Work out the finished part from the listing and answer in its coordinate system (mm). A direction names the side the tool comes from. Give positions to 0.01 mm unless a question says otherwise; leave off trailing zeros. Order: outer loops, then holes, each group sorted by start corner. A loop starts at its lowest first (then second) coordinate and runs counter-clockwise, first axis right, second up. Notation, with made-up numbers: (73, 72) -> (128, 72) arc R19 cw to (128, 92) -> close; hole circle Ø9 at (19, 58). An arc over 180 degrees is marked (long way). Use a Markdown table: item, result. Add a question column.
```python
from build123d import *

# Parameters (mm, degrees)
SKETCH_1_R            = 13.5
EXTRUDE_1_DEPTH       = 8
SKETCH_7_W            = 34
SKETCH_7_H            = 30
SKETCH_7_R            = 13.5
EXTRUDE_2_DEPTH       = 8
SKETCH_11_W           = 5
SKETCH_11_H           = 30
EXTRUDE_6_DEPTH       = 40
FILLET_2_R            = 10
SKETCH_13_R           = 8.5
SKETCH_13_R_2         = 7.5
CUT_EXTRUDE_3_DEPTH   = 2.5
SKETCH_14_R           = 3.5
CUT_EXTRUDE_4_DEPTH   = 36
SKETCH_22_W           = 41
SKETCH_22_H           = 5
EXTRUDE_8_DEPTH       = 8
SKETCH_23_W           = 12
SKETCH_23_H           = 8
CUT_EXTRUDE_6_DEPTH   = 20
RIB_1_REACH           = 62.671
SKETCH_24_WALL_W      = 135.42553647
SKETCH_24_WALL_H      = 5
EXTRUDE_9_DEPTH       = 4
F_3_0MM_1_D           = 3
F_3_0MM_1_CSINK_D     = 3.05
F_3_0MM_1_CSINK_ANGLE = 90
SKETCH_27_W           = 14.5
SKETCH_27_H           = 20
EXTRUDE_10_DEPTH      = 8
F_3_0MM_2_D           = 3
F_3_0MM_2_CSINK_D     = 3.05
F_3_0MM_2_CSINK_ANGLE = 90
CHAMFER_5_SIZE        = 3
SKETCH_29_R           = 12.5
SKETCH_29_R_2         = 10
EXTRUDE_11_DEPTH      = 5.5
CHAMFER_4_SIZE        = 0.5


with BuildPart() as part:
    # 草图1 → 凸台-拉伸1 (new body)
    with BuildSketch(Plane(origin=(0, 0, 0), x_dir=(1, 0, 0), z_dir=(0, 1, 0))):
        with Locations(Location((0, 0, 0), (0, 0, 270))):
            Circle(SKETCH_1_R)
    extrude(amount=EXTRUDE_1_DEPTH)

    # 草图7 → 凸台-拉伸2 (add)
    with BuildSketch(Plane.XZ):
        Rectangle(SKETCH_7_W, SKETCH_7_H)
        Circle(SKETCH_7_R, mode=Mode.SUBTRACT)
    extrude(amount=-EXTRUDE_2_DEPTH)

    # 草图11 → 凸台-拉伸6 (add)
    with BuildSketch(Plane.XZ):
        with Locations((-18.5, 0)):
            Rectangle(SKETCH_11_W, SKETCH_11_H)
        with Locations((17.5, 0)):
            Rectangle(SKETCH_11_W, SKETCH_11_H)
    extrude(amount=-EXTRUDE_6_DEPTH)

    # 圆角2
    fillet_2_edges = [part.edges().sort_by_distance(p)[0] for p in [
        (-18.5, 40, -15),
        (-18.5, 40, 15),
        (17.5, 40, 15),
        (17.5, 40, -15),
    ]]
    fillet(fillet_2_edges, radius=FILLET_2_R)

    # 草图13 → 切除-拉伸3 (cut)
    with BuildSketch(Plane(origin=(20, 0, 0), x_dir=(0, 0, -1), z_dir=(1, 0, 0))):
        with Locations((0, 22.5)):
            Circle(SKETCH_13_R)
        with Locations((0, 22.5)):
            Circle(SKETCH_13_R_2, mode=Mode.SUBTRACT)
    cut_extrude_3 = extrude(amount=-CUT_EXTRUDE_3_DEPTH, mode=Mode.SUBTRACT)

    # 草图14 → 切除-拉伸4 (cut)
    with BuildSketch(Plane(origin=(20, 0, 0), x_dir=(0, 0, -1), z_dir=(1, 0, 0))):
        with Locations((0, 22.5)):
            Circle(SKETCH_14_R)
    cut_extrude_4 = extrude(amount=-CUT_EXTRUDE_4_DEPTH, mode=Mode.SUBTRACT)

    # 草图22 → 凸台-拉伸8 (add)
    with BuildSketch(Plane.XZ):
        with Locations((-0.5, -17.5)):
            Rectangle(SKETCH_22_W, SKETCH_22_H)
    extrude(amount=-EXTRUDE_8_DEPTH)

    # 草图23 → 切除-拉伸6 (cut)
    with BuildSketch(Plane.XY.offset(15)):
        with Locations((-0.5, 4)):
            Rectangle(SKETCH_23_W, SKETCH_23_H)
    extrude(amount=-CUT_EXTRUDE_6_DEPTH, mode=Mode.SUBTRACT)

    # 草图24 wall → 筋1 (add, up to next)
    with BuildSketch(Plane(origin=(-21, 13.5, -17.5), x_dir=(0, 0.910366477463, 0.413802944301), z_dir=(0, 0.413802944301, -0.910366477463)), mode=Mode.PRIVATE) as rib_1_sk1:
        with Locations((0, 2.5)):
            Rectangle(SKETCH_24_WALL_W, SKETCH_24_WALL_H)
    rib_1_tool1 = extrude(rib_1_sk1.sketch, amount=-RIB_1_REACH, mode=Mode.PRIVATE) - part.part
    add(rib_1_tool1.solids().sort_by_distance((-21, 13.5, -17.5))[0])

    # 草图25 → 凸台-拉伸9 (add)
    with BuildSketch(Plane(origin=(20, 0, 0), x_dir=(0, 0, -1), z_dir=(1, 0, 0))):
        Polygon((20, 8), (15, 19), (15, 8), align=None)
    extrude(amount=-EXTRUDE_9_DEPTH)

    # Ø3.0mm 暗销孔1 (through all)
    with Locations(Plane(origin=(20, 3, 11), x_dir=(0, 0, 1), z_dir=(1, 0, 0))):
        with Locations((0, 0), (-12, 0)):
            CounterSinkHole(F_3_0MM_1_D / 2, F_3_0MM_1_CSINK_D / 2, counter_sink_angle=F_3_0MM_1_CSINK_ANGLE)

    # 草图27 → 凸台-拉伸10 (add)
    with BuildSketch(Plane.XZ):
        with Locations((-13.75, 5)):
            Rectangle(SKETCH_27_W, SKETCH_27_H)
        with Locations((12.75, 5)):
            Rectangle(SKETCH_27_W, SKETCH_27_H)
    extrude(amount=EXTRUDE_10_DEPTH)

    # Ø3.0mm 暗销孔2 (through all)
    with Locations(Plane(origin=(20, -4.999960937, 11), x_dir=(0, 0, 1), z_dir=(1, 0, 0))):
        with Locations((0, 0), (-12, 0)):
            CounterSinkHole(F_3_0MM_2_D / 2, F_3_0MM_2_CSINK_D / 2, counter_sink_angle=F_3_0MM_2_CSINK_ANGLE)

    # 倒角5
    chamfer_5_edges = [part.edges().sort_by_distance(p)[0] for p in [
        (-0.5, 0, -20),
        (-11.25, 8, 15),
        (-13.75, 0, -5),
        (-13.75, -8, -5),
        (-13.75, -8, 15),
        (12.75, 0, -5),
        (12.75, -8, 15),
        (12.75, -8, -5),
        (10.25, 8, 15),
    ]]
    chamfer(chamfer_5_edges, length=CHAMFER_5_SIZE)

    # 草图29 → 凸台-拉伸11 (add)
    with BuildSketch(Plane.ZY.offset(-15)):
        with Locations((0, 22.5)):
            Circle(SKETCH_29_R)
        with Locations((0, 22.5)):
            Circle(SKETCH_29_R_2, mode=Mode.SUBTRACT)
    extrude_11 = extrude(amount=EXTRUDE_11_DEPTH)

    # 镜向1: 切除-拉伸3, 切除-拉伸4, 凸台-拉伸11 across plane
    add(cut_extrude_3.mirror(Plane.ZY.offset(0.5)), mode=Mode.SUBTRACT)
    add(cut_extrude_4.mirror(Plane.ZY.offset(0.5)), mode=Mode.SUBTRACT)
    add(extrude_11.mirror(Plane.ZY.offset(0.5)))

    # 倒角4
    chamfer_4_edges = [part.edges().sort_by_distance(p)[0] for p in [
        (9.5, 22.5, -12.5),
        (9.5, 22.5, -10),
        (-21, 22.5, 3.5),
        (-10.5, 22.5, -12.5),
        (-10.5, 22.5, -10),
        (20, 22.5, 3.5),
    ]]
    chamfer(chamfer_4_edges, length=CHAMFER_4_SIZE)


solid = part.part
```
1) Which of the six approach directions +Z, -Z, +X, -X, +Y, -Y give full straight-line access (tool end or side, diameter ignored) to faces 1 (the cylindrical face through (-19.768, 29.936, 0.976)), 2 (the cylindrical face through (-18.46, 37.15, -11.99))?
2) Determine the mould class of faces 3 (the flat face through (16, 11, -16)), 4 (the cylindrical face through (12.535, 10.297, -2.71)), 5 (the flat face through (-14, -7, 13)), 6 (the flat face through (20, 26, 3)) for opening direction X: released by +X, released by -X, zero draft, split by the parting line, or undercut.
3) Straight lines are drawn through the part: line 1 (Y direction, x = 16, z = 0); line 2 (X direction, y = 25.5, z = -8.5); line 3 (Y direction, x = -10, z = 0). For each, find the intervals that lie inside material, in ascending order.
4) The part is cut by section B-B, the plane y = 22.5. State how many separate pieces and enclosed holes the cut face has, then the cut area to 4 significant figures.
5) The part is cut by section C-C, the plane x = -9.5. Determine the outline of the cut face in (y, z).
6) Flat-ended cylindrical pins translate along their axes: pin 1 (2 mm diameter, centred on x = 8, z = -8.5, fed in from -Y); pin 2 (1.5 mm diameter, centred on y = -2, z = -10.5, fed in from +X); pin 3 (5.5 mm diameter, centred on x = 18, y = 23.5, fed in from -Z). Find the tip coordinate at first contact, or state that the pin passes through.
7) The part is cut by section A-A, the plane x = 12.5. Determine the outline of the cut face in (y, z), then the cut area to 3 significant figures.
A:
| question | item | result |
|---|---|---|
| 1 | face 1 | -X |
| 1 | face 2 | -Z, +X, -X, +Y |
| 2 | face 3 | undercut |
| 2 | face 4 | undercut |
| 2 | face 5 | zero draft |
| 2 | face 6 | released by +X |
| 3 | line 1 | -8 to -6.12, -3.88 to 1.88, 4.12 to 19, 26 to 40 |
| 3 | line 2 | -21 to -16, 15 to 20 |
| 3 | line 3 | -8 to -6.12, -3.88 to 1.88, 4.12 to 8 |
| 4 | separate pieces | 4 |
| 4 | enclosed holes | 0 |
| 4 | area | 273.5 mm^2 |
| 5 | outline | (-8, -2) -> (-5, -5) -> (-3, -5) -> (0, -8) -> (0, -17) -> (3, -20) -> (8, -20) -> (8, 12) -> (5, 15) -> (-5, 15) -> (-8, 12) -> close; hole circle Ø3 at (-5, -1); hole circle Ø3 at (-5, 11); hole circle Ø3 at (3, -1); hole circle Ø3 at (3, 11) |
| 6 | pin 1 | y = -0.5 |
| 6 | pin 2 | through |
| 6 | pin 3 | z = -15 |
| 7 | outline | (-8, -2) -> (-5, -5) -> (-3, -5) -> (0, -8) -> (0, -17) -> (3, -20) -> (8, -20) -> (8, 12) -> (5, 15) -> (-5, 15) -> (-8, 12) -> close; circle Ø25 at (22.5, 0); hole circle Ø3 at (-5, -1); hole circle Ø3 at (-5, 11); hole circle Ø3 at (3, -1); hole circle Ø3 at (3, 11); hole circle Ø20 at (22.5, 0) |
| 7 | area | 575 mm^2 |
